Read the model definition and answer for the solid it produces. Units are mm, in the model's axes. A direction names the side the tool comes from. Give positions to 0.01 mm unless a question says otherwise; leave off trailing zeros. Write each loop counter-clockwise with the first axis right and the second up, starting at its lowest first coordinate (ties: lowest second). Pieces come first, ordered by that corner, then holes.
Autodesk Inventor part; units mm, degrees
ref_plane "YZ Plane" through (0, 0, 0) normal (1, 0, 0) x (0, 1, 0)
ref_plane "XZ Plane" through (0, 0, 0) normal (0, 1, 0) x (-1, 0, 0)
ref_plane "XY Plane" through (0, 0, 0) normal (0, 0, 1) x (1, 0, 0)
sketch "Sketch1" plane through (0, 0, 0) normal (0, 0, 1) x (1, 0, 0)
  line L0 (0, 0) -> (300, 0)
  line L1 (300, 0) -> (300, 200)
  line L2 (300, 200) -> (0, 200)
  line L3 (0, 200) -> (0, 0)
  dimension "d0" = 200
  dimension "d1" = 300
extrude "Extrusion1" add sketch "Sketch1" along normal blind 90
sketch "Sketch2" plane through (0, 0, 0) normal (0, 0, -1) x (-1, 0, 0)
  line L0 (-10, 10) -> (-290, 10)
  line L1 (-290, 10) -> (-290, 190)
  line L2 (-290, 190) -> (-10, 190)
  line L3 (-10, 190) -> (-10, 10)
  line L4 (0, 0) -> (-300, 0)
  line L5 (0, 200) -> (0, 0)
  dimension "d4" = 180
  dimension "d5" = 280
  dimension "d6" = 10
  dimension "d7" = 10
extrude "Extrusion2" cut sketch "Sketch2" against normal blind 80
sketch "Sketch4" plane through (0, 0, 0) normal (0, 0, -1) x (-1, 0, 0)
  circle A0 centre (-6.4515, 6.4515) radius 1.4515
  circle A1 centre (-6.4515, 193.5485) radius 1.4515
  circle A2 centre (-293.5485, 193.5485) radius 1.4515
  circle A3 centre (-293.5485, 6.4515) radius 1.4515
  line L0 (0, 0) -> (-300, 0)
  line L1 (0, 200) -> (0, 0)
  line L2 (-300, 200) -> (0, 200)
  line L3 (-300, 0) -> (-300, 200)
  dimension "d18" = 2.903
  dimension "d19" = 2.903
  dimension "d20" = 2.903
  dimension "d21" = 2.903
  dimension "d22" = 5
  dimension "d23" = 5
  dimension "d24" = 5
  dimension "d25" = 5
  dimension "d26" = 5
  dimension "d27" = 5
  dimension "d28" = 5
  dimension "d29" = 5
extrude "Extrusion4" cut sketch "Sketch4" against normal blind 17 contours A0 | A1 | A2 | A3
sketch "Sketch5" plane through (0, 0, 0) normal (0, -1, 0) x (1, 0, 0)
  circle A0 centre (265, 55) radius 4
  circle A1 centre (35, 55) radius 4
  line L0 (0, 90) -> (300, 90)
  line L1 (300, 0) -> (300, 90)
  line L2 (0, 0) -> (0, 90)
  dimension "d32" = 8
  dimension "d33" = 8
  dimension "d34" = 35
  dimension "d35" = 35
  dimension "d36" = 35
  dimension "d37" = 35
extrude "Extrusion5" cut sketch "Sketch5" against normal through all
sketch "Sketch6" plane through (0, 0, 80) normal (0, 0, -1) x (-1, 0, 0)
  point P0 (0, 0)
sketch "Sketch7" plane through (0, 0, 80) normal (0, 0, -1) x (-1, 0, 0)
  line L0 (-10, 190) -> (-10, 10)
  point P0 (0, 0)
sketch "Sketch8" plane through (0, 0, 0) normal (-1, 0, 0) x (0, 0, 1)
  circle A0 centre (45, 100) radius 2.5
  line L0 (0, 0) -> (90, 0)
  line L1 (0, 200) -> (0, 0)
  dimension "d57" = 5
  dimension "d58" = 100
  dimension "d59" = 45
extrude "Extrusion6" cut sketch "Sketch8" against normal blind 10
equation "\"BendRadius\" = Thickness"
equation "\"BendReliefWidth\" = Thickness"
equation "\"BendReliefDepth\" = 0.5 * Thickness"
equation "\"CornerReliefSize\" = 4 * Thickness"
equation "\"MinimumRemnant\" = 2 * Thickness"
equation "\"TransitionRadius\" = BendRadius"
equation "\"JacobiRadiusSize\" = BendRadius"
equation "\"GapSize\" = Thickness"
properties part number "base"
Item 1: Section B-B (x = 265) is taken. Write down the section's boundary in (y, z), and give its area (3 significant figures).
Result set:
outline: (0, 0) - (10, 0) - (10, 51) - (0, 51) - close; (0, 59) - (10, 59) - (10, 80) - (190, 80) - (190, 59) - (200, 59) - (200, 90) - (0, 90) - close; (190, 0) - (200, 0) - (200, 51) - (190, 51) - close
area: 3,440 mm2
Item 2: This flat-tipped pin is pushed along its axis until it touches: pin 1 Ø0.9 at (x, y) = (293, 6.5) entering from -Z. Where does it stop, or does it pass through?
Result set:
pin 1: stops at z = 17
Item 3: Which of the six approach directions +Z, -Z, +X, -X, +Y, -Y give full straight-line access (tool end or side, diameter ignored) to faces 1 (the flat face through (138, 4, 0)), 2 (the flat face through (152, 190, 39))?
Result set:
face 1: -Z, +X, -X, +Y, -Y
face 2: -Z
Item 4: Section C-C (y = 92) is taken. Write down the section's boundary in (x, z), and give its area (3 significant figures).
Result set:
outline: (0, 0) - (10, 0) - (10, 80) - (290, 80) - (290, 0) - (300, 0) - (300, 90) - (0, 90) - close
area: 4,600 mm2
Item 5: Find the intervals of material crossed by line 1 along Z through (x, y) = (265, 4); line 2 along X through (y, z) = (44, 36); line 3 along Y through (x, z) = (224, 66), in increasing order.
Result set:
line 1: z = 0 to 51, 59 to 90
line 2: x = 0 to 10, 290 to 300
line 3: y = 0 to 10, 190 to 200
Item 6: Determine the mould class of faces 3 (the flat face through (152, 101, 80)), 4 (the cylindrical face through (34.133, 4.93, 51.095)), 5 (the flat face through (148, 0, 44)) for opening direction Z: pulls with the +Z half, pulls with the -Z half, needs draft (parallel to the pull), parting line crosses it, or undercut.
Result set:
face 3: pulls with the -Z half
face 4: undercut
face 5: needs draft
Item 7: Section A-A (z = 55) is taken. Write down the section's boundary in (x, y), and give its area (3 significant figures).
Result set:
outline: (0, 0) - (31, 0) - (31, 10) - (10, 10) - (10, 190) - (31, 190) - (31, 200) - (0, 200) - close; (39, 0) - (261, 0) - (261, 10) - (39, 10) - close; (39, 190) - (261, 190) - (261, 200) - (39, 200) - close; (269, 0) - (300, 0) - (300, 200) - (269, 200) - (269, 190) - (290, 190) - (290, 10) - (269, 10) - close
area: 9,280 mm2
Item 8: Section D-D (z = 11) is taken. Write down the section's boundary in (x, y), and give its area (3 significant figures).
Result set:
outline: (0, 0) - (300, 0) - (300, 200) - (0, 200) - close; hole circle Ø2.9 at (6.45, 6.45); hole circle Ø2.9 at (6.45, 193.55); hole (10, 10) - (290, 10) - (290, 190) - (10, 190) - close; hole circle Ø2.9 at (293.55, 6.45); hole circle Ø2.9 at (293.55, 193.55)
area: 9,570 mm2
